Work out the finished part from the listing and answer in its coordinate system (mm). Coordinates: 2 decimals unless noted, no trailing zeros. Loops run counter-clockwise (first coordinate to the right, second up) from the corner with the lowest first, then second, coordinate; pieces in that order, holes last. Notation, with made-up numbers: (70.5, 67.5) -> (106.5, 67.5) arc R18 ccw to (106.5, 88.5) -> close; hole circle Ø7 at (87.25, -12). An arc over 180 degrees is marked (long way). Use a Markdown table: item, result. Add a question column.
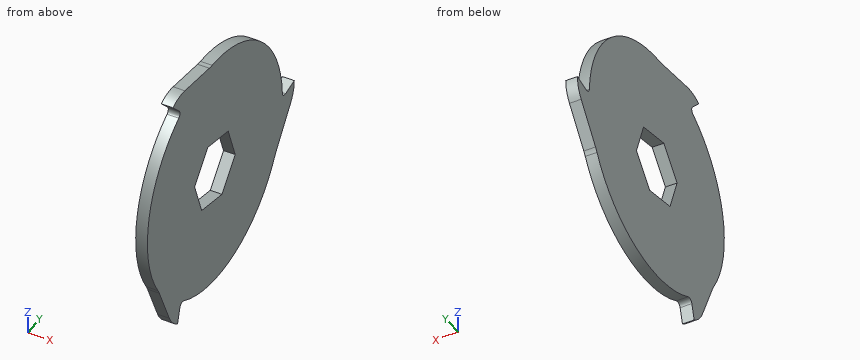
```python
from build123d import *

# Parameters (mm, degrees)
SKETCH1_R         = 51
EXTRUDE1_DEPTH    = 2.5
EXTRUDE2_DEPTH    = 2.5
CIRPATTERN1_COUNT = 3


with BuildPart() as part:
    # Sketch1 → Extrude1 (new, symmetric)
    with BuildSketch(Plane(origin=(0, 0, 0), x_dir=(0, 0, -1), z_dir=(1, 0, 0))):
        Circle(SKETCH1_R)
        Polygon((14.648358264, 5.331566389), (2.706907197, 15.351633575), (-11.941451067, 10.020067186), (-14.648358264, -5.331566389), (-2.706907197, -15.351633575), (11.941451067, -10.020067186), align=None, mode=Mode.SUBTRACT)
    extrude(amount=EXTRUDE1_DEPTH, both=True)

    # Sketch2 → Extrude2 (add, symmetric)
    with BuildSketch(Plane(origin=(0, 0, 0), x_dir=(0, 0, -1), z_dir=(1, 0, 0))):
        with BuildLine():
            Line((-2, 59.956265369), (-0.262596806, 53.472188376))
            ThreePointArc((-0.262596806, 53.472188376), (-0.582870999, 51.770144067), (-2.111639083, 50.956265369))
            ThreePointArc((-2.111639083, 50.956265369), (11.148765219, 49.766505142), (23.649399595, 45.185239833))
            ThreePointArc((23.649399595, 45.185239833), (22.732801751, 45.706819988), (21.855117489, 46.291514612))
            Line((21.855117489, 46.291514612), (6.74998787, 57.139767012))
            ThreePointArc((6.74998787, 57.139767012), (2.596056753, 59.234789884), (-2, 59.956265369))
        make_face()
    extrude2 = extrude(amount=EXTRUDE2_DEPTH, both=True)

    # CirPattern1: Extrude2 ×3 about axis
    cirpattern1_axis = Axis((0, 0, 0), (1, 0, 0))
    for i in range(1, CIRPATTERN1_COUNT):
        add(extrude2.rotate(cirpattern1_axis, i * 360 / CIRPATTERN1_COUNT))


solid = part.part
```
Item 1: Find the intervals of material crossed by probe 1 along Z at (x, y) = (1.2, -9); probe 2 along Z at (x, y) = (2.25, 10); probe 3 along Y at (x, z) = (-0.65, 11), in increasing order.
Item 2: Section A-A (z = -4.5) is taken. Determine the outline of the cut face in (x, y).
Item 3: Section B-B (y = 13) is taken. Determine the outline of the cut face in (x, z), then the cut area to 3 significant figures.
Item 4: Given pin 1 (2 mm diameter, centred on x = 1.5, z = -13, fed in from +Y); pin 2 (1 mm diameter, centred on x = 1.5, z = 35.5, fed in from +Y), each flat-ended and moving along its own axis, determine where each tip first touches the part or whether it passes through.
Item 5: Section C-C (x = 1.4) is taken. Determine the outline of the cut face in (y, z), then the cut area to 3 significant figures.
Item 6: Section D-D (z = -33) is taken. Determine the outline of the cut face in (x, y).
Output:
| question | item | result |
|---|---|---|
| 1 | probe 1 | z = -50.2 to -12.12, 10.28 to 51.49 |
| 1 | probe 2 | z = -50.01 to -9.08, 11.94 to 50.01 |
| 1 | probe 3 | y = -49.8 to -8.39, 10.36 to 49.8 |
| 2 | outline | (-2.5, -50.8) -> (2.5, -50.8) -> (2.5, -12.73) -> (-2.5, -12.73) -> close; (-2.5, 13.85) -> (2.5, 13.85) -> (2.5, 58.47) -> (-2.5, 58.47) -> close |
| 3 | outline | (-2.5, -49.32) -> (2.5, -49.32) -> (2.5, -5.51) -> (-2.5, -5.51) -> close; (-2.5, 3.75) -> (2.5, 3.75) -> (2.5, 49.32) -> (-2.5, 49.32) -> close |
| 3 | area | 447 mm2 |
| 4 | pin 1 | stops at y = 53.37 |
| 4 | pin 2 | stops at y = 37.09 |
| 5 | outline | (-43.07, -27.31) arc R15 cw to (-42.07, -29.16) -> (-34.42, -46.11) arc R15 ccw to (-28.25, -52.92) -> (-26.51, -46.44) arc R2 cw to (-23.65, -45.19) arc R51 ccw to (45.19, -23.65) arc R15 cw to (46.29, -21.86) -> (57.14, -6.75) arc R15 ccw to (59.96, 2) -> (53.47, 0.26) arc R2 cw to (50.96, 2.11) arc R51 ccw to (-2.11, 50.96) arc R15 cw to (-4.22, 51.02) -> (-22.72, 52.86) arc R15 ccw to (-31.71, 50.92) -> (-26.96, 46.18) arc R2 cw to (-27.31, 43.07) arc R51 ccw to start; hole (-15.35, 2.71) -> (-10.02, -11.94) -> (5.33, -14.65) -> (15.35, -2.71) -> (10.02, 11.94) -> (-5.33, 14.65) -> close |
| 5 | area | 7,860 mm2 |
| 6 | outline | (-2.5, -40.34) -> (2.5, -40.34) -> (2.5, 38.88) -> (-2.5, 38.88) -> close |
